Design review of the part shown in the three views and the two pictorial views. Dimensions are in mm from the part's minimum x, y and z. A direction names the side the tool comes from. Round coordinates to 2 decimals unless told otherwise and drop trailing zeros. Loops run counter-clockwise (first coordinate to the right, second up) from the corner with the lowest first, then second, coordinate; pieces in that order, holes last. Notation, with made-up numbers: (46, 29) -> (81, 29) arc R4 ccw to (81, 34) -> close; hole circle Ø2 at (-24.5, -27). An arc over 180 degrees is marked (long way). Use CSV: the item, a comma, the result in double quotes. Start each with the question number.
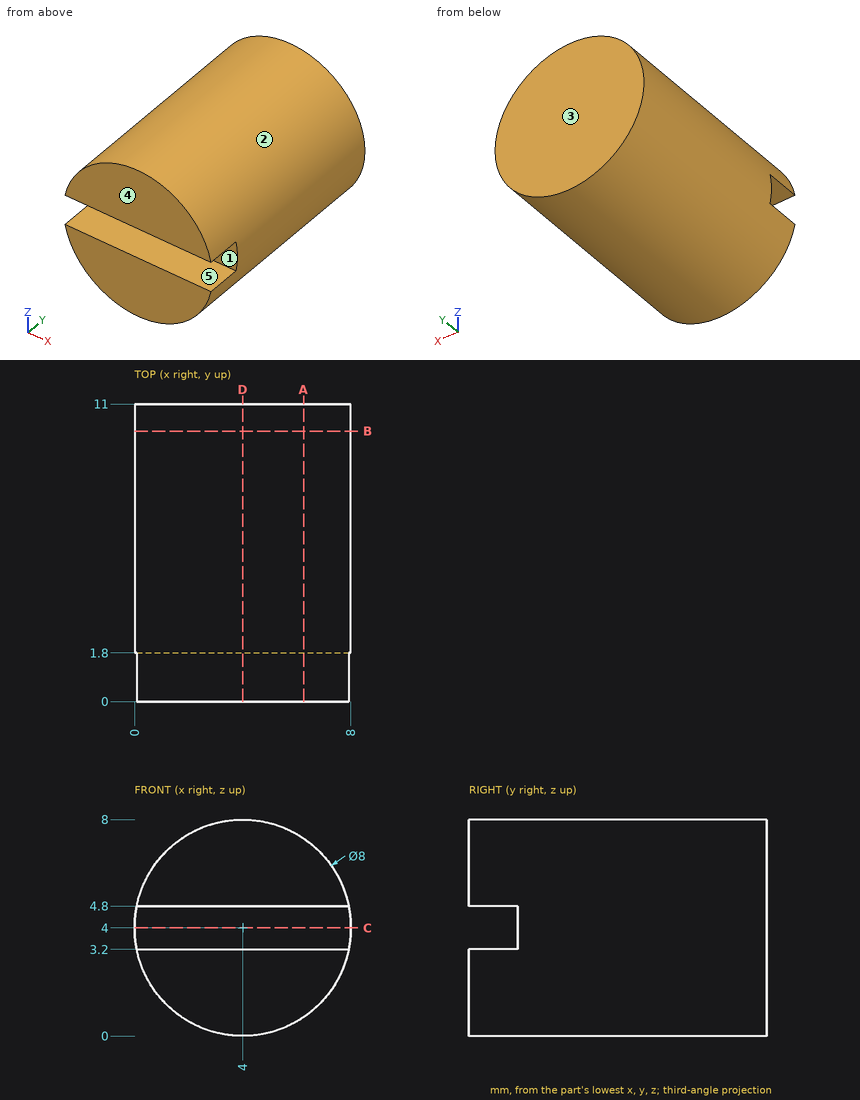
1. Take a section at D-D, the plane x = 4. Give the boundary of the cut face in (y, z).
2. Take a section at C-C, the plane z = 4. Give the boundary of the cut face in (x, y).
3. For line 1 along Z through (x, y) = (5.25, 0.5); line 2 along Z through (x, y) = (7, 0.5); line 3 along Y through (x, z) = (6.5, 3.25), list the stretches that pass through material, from the lowest coordinate up. Write a range as from..to.
4. For the marked faces 4 and 5, list the 3-axis set-ups (+Z, -Z, +X, -X, +Y, -Y) from which the entire face can be reached by the end or side of a thin tool; tool diameter is ignored.
5. The part is to be moulded in two halves that separate along Z. For the marked faces 1, 2 and 3, say which applies: pulls with the +Z half, pulls with the -Z half, needs draft (parallel to the pull), parting line crosses it, or undercut.
6. Take a section at A-A, the plane x = 6.25. Give the boundary of the cut face in (y, z).
7. Clearance check with flat-ended pins moving along their axes: P1, Ø1.5, axis at x = 6, y = 6.5, coming from the +Z side; P2, Ø0.5, axis at x = 3.5, z = 4, coming from the -Y side; P3, Ø1.5, axis at y = 5.5, z = 3, coming from the +X side. State where each tip first meets the part, or that it passes through.
8. Take a section at B-B, the plane y = 10. Give the boundary of the cut face in (x, z).
Results:
1,outline,"(0, 0) -> (11, 0) -> (11, 8) -> (0, 8) -> (0, 4.8) -> (1.8, 4.8) -> (1.8, 3.2) -> (0, 3.2) -> close"
2,outline,"(0, 1.8) -> (8, 1.8) -> (8, 11) -> (0, 11) -> close"
3,line 1,"0.2..3.2, 4.8..7.8"
3,line 2,"1.35..3.2, 4.8..6.65"
3,line 3,"1.8..11"
4,face 4,"+Z, -Z, +X, -X, -Y"
4,face 5,"+X, -X, -Y"
5,face 1,"undercut"
5,face 2,"parting line crosses it"
5,face 3,"needs draft"
6,outline,"(0, 0.69) -> (11, 0.69) -> (11, 7.31) -> (0, 7.31) -> (0, 4.8) -> (1.8, 4.8) -> (1.8, 3.2) -> (0, 3.2) -> close"
7,P1,"z = 7.8"
7,P2,"y = 1.8"
7,P3,"x = 7.99"
8,outline,"circle Ø8 at (4, 4)"
